Autodesk Fusion 360 part; units mm, degrees
sketch "Sketch1" plane through (0, 0, 0) normal (0, 0, 1) x (1, 0, 0)
  circle A0 centre (0, 0) radius 100
  dimension "d1" = 200
extrude "Extrude1" add sketch "Sketch1" along normal blind 75
chamfer "Chamfer1" distance 10 angle 45 1 edges at (-93.2327, -36.1615, 75)
sketch "Sketch2" plane through (0, 0, 75) normal (0, 0, 1) x (-1, 0, 0)
  circle A0 centre (0, 0) radius 90
  circle A1 centre (0, 0) radius 100
  line L0 (0, 0) -> (0, 100)
  line L1 (0, 0) -> (100, 0)
  circle A2 centre (0, 0) radius 80
  line L2 (0, 0) -> (100, 0)
  line L3 (0, 0) -> (139.8681, 80.7529)
  line L4 (0, 0) -> (161.5058, 0) construction
  line L5 (0, 0) -> (61.5265, 106.567)
  dimension "d5" = 160
  dimension "d6" = 30
  dimension "d7" = 60
extrude "Extrude2" cut sketch "Sketch2" against normal blind 60 contours A0 A2 L3 L5 | A0 A1 L3 L5
sketch "Sketch3" plane through (0, 0, 75) normal (0, 0, 1) x (-1, 0, 0)
  line L0 (40, 69.282) -> (45, 77.9423)
  arc A0 (45, 77.9423) -> (77.9423, 45) centre (0, 0) ccw
  line L1 (77.9423, 45) -> (69.282, 40)
  arc A1 (69.282, 40) -> (40, 69.282) centre (0, 0) ccw
  circle A2 centre (0, 0) radius 60
  dimension "d11" = 120
extrude "Extrude3" add sketch "Sketch3" along normal blind 9 draft -45 contours A2
sketch "Sketch4" plane through (0, 0, 84) normal (0, 0, 1) x (-1, 0, 0)
  circle A0 centre (0, 0) radius 51
  circle A1 centre (0, 0) radius 15
  dimension "d14" = 30
extrude "Extrude4" add sketch "Sketch4" along normal blind 20 contours A1
Could you check a few things on this model? Use its own coordinates, in mm. A direction names the side the tool comes from. Coordinates: 2 decimals unless noted, no trailing zeros. Loops run counter-clockwise (first coordinate to the right, second up) from the corner with the lowest first, then second, coordinate; pieces in that order, holes last.
1. Imagine slicing it at D-D (z = 17.5). Please give me the cut outline in (x, y).
2. I need wall thicknesses on L1, parallel to Z at x = 34, y = -81; L2, parallel to Y at x = -41.5, z = 36; L3, parallel to Z at x = 12, y = -45.5. Which ranges of each line are inside material? Lowest first, please.
3. For P1, Ø2, axis at x = -6.5, z = 19, coming from the +Y side; P2, Ø8, axis at x = -73, z = 26, coming from the +Y side; P3, Ø1, axis at x = 44, y = 73, coming from the +Z side, each with a flat end and sliding along its axis, tell me the tip position at first contact or that it passes through.
4. For faces 1 (the face through (-77.82, -44.93, 45.42)), 2 (the face through (-1, 1, 0)), 3 (the face through (-44.93, -77.82, 45.42)), 4 (the face through (-11, 11, 84)), which set-ups out of +Z, -Z, +X, -X, +Y, -Y let a thin tool reach every point of the face, with its end or its side?
5. Imagine slicing it at A-A (y = 0). Please give me the cut outline in (x, z).
6. Imagine slicing it at C-C (z = 94). Please give me the cut outline in (x, y).
7. We'd pull the mould along X, two halves only. Please class faces 5 (the face through (0, 0, 104)), 6 (the face through (14.985, 0.66, 93.86)), 7 (the face through (-56.775, -56.361, 45.42)): released by +X, released by -X, zero draft, split by the parting line, or undercut.
Computed values:
1. outline: (-86.6, -50) - (-69.28, -40) arc R80 ccw to (-40, -69.28) - (-50, -86.6) arc R100 ccw (long way) to start
2. L1: z = 0 to 75
2. L2: y = -90.98 to -71.88, -68.39 to 90.98
2. L3: z = 0 to 84
3. P1: stops at y = 99.85
3. P2: stops at y = 72.38
3. P3: stops at z = 75
4. face 1: +Z, -Y
4. face 2: -Z, +X, -X, +Y, -Y
4. face 3: +Z, -X
4. face 4: +Z
5. outline: (-100, 0) - (100, 0) - (100, 65) - (90, 75) - (60, 75) - (51, 84) - (15, 84) - (15, 104) - (-15, 104) - (-15, 84) - (-51, 84) - (-60, 75) - (-90, 75) - (-100, 65) - close
6. outline: circle Ø30 at (0, 0)
7. face 5: zero draft
7. face 6: split by the parting line
7. face 7: undercut
